Check sheet for the modelled part. Datum: model origin and axes. Units: mm. A direction names the side the tool comes from. Give positions to 0.01 mm unless a question says otherwise; leave off trailing zeros. Loops run counter-clockwise (first coordinate to the right, second up) from the corner with the lowest first, then second, coordinate; pieces in that order, holes last. Notation, with made-up numbers: M -17,81.5 L 38,81.5 A21 ccw 38,116.5 Z; hole C 71,74 d2. An arc over 180 degrees is marked long. Use one line per item in the form item = value.
from build123d import *

# Parameters (mm, degrees)
SKETCH1_W                 = 140
SKETCH1_H                 = 30
BOSS_EXTRUDE1_DEPTH       = 5
EXTRUDE_THIN1_START       = -5
EXTRUDE_THIN1_OUTLINE_W   = 20
EXTRUDE_THIN1_OUTLINE_H   = 30
EXTRUDE_THIN1_OUTLINE_W_2 = 16
EXTRUDE_THIN1_OUTLINE_H_2 = 26
EXTRUDE_THIN1_DEPTH       = 85
FILLET1_SIZE              = 15
SKETCH3_R                 = 17
SKETCH3_R_2               = 15
EXTRUDE_THIN2_DEPTH       = 40
SKETCH4_W                 = 35
SKETCH4_H                 = 24.79
BOSS_EXTRUDE2_DEPTH       = 160


with BuildPart() as part:
    # Sketch1 → Boss-Extrude1 (new body)
    with BuildSketch(Plane(origin=(0, 0, 0), x_dir=(1, 0, 0), z_dir=(0, 1, 0))):
        Rectangle(SKETCH1_W, SKETCH1_H)
    extrude(amount=-BOSS_EXTRUDE1_DEPTH)

    # Extrude-Thin1: read off the stored shape, not the designer's step
    # Extrude-Thin1 outline → Extrude-Thin1 (add)
    # profile 1 of 2: a face of its own
    with BuildSketch(Plane(origin=(0, 0, 0), x_dir=(1, 0, 0), z_dir=(0, 1, 0)).offset(EXTRUDE_THIN1_START)):
        with Locations((60, 0)):
            Rectangle(EXTRUDE_THIN1_OUTLINE_W, EXTRUDE_THIN1_OUTLINE_H)
        with Locations((60, 0)):
            Rectangle(EXTRUDE_THIN1_OUTLINE_W_2, EXTRUDE_THIN1_OUTLINE_H_2, mode=Mode.SUBTRACT)
    # profile 2 of 2: a face of its own
    with BuildSketch(Plane(origin=(0, 0, 0), x_dir=(1, 0, 0), z_dir=(0, 1, 0)).offset(EXTRUDE_THIN1_START)):
        with Locations((-60, 0)):
            Rectangle(EXTRUDE_THIN1_OUTLINE_W, EXTRUDE_THIN1_OUTLINE_H)
        with Locations((-60, 0)):
            Rectangle(EXTRUDE_THIN1_OUTLINE_W_2, EXTRUDE_THIN1_OUTLINE_H_2, mode=Mode.SUBTRACT)
    extrude(amount=EXTRUDE_THIN1_DEPTH)

    # Fillet1
    # a fillet whose section is not a circle: 15 mm, written as the material it takes off along each edge
    with BuildSketch(Plane(origin=(-107.5, 80, 15), x_dir=(0, -1, 0), z_dir=(1, 0, 0)), Plane(origin=(-12.5, 80, -15), x_dir=(0, -1, 0), z_dir=(-1, 0, 0)), Plane(origin=(107.5, 80, -15), x_dir=(0, -1, 0), z_dir=(-1, 0, 0)), Plane(origin=(12.5, 80, 15), x_dir=(0, -1, 0), z_dir=(1, 0, 0))) as fillet1_piece_1:
        with BuildLine():
            Bezier((FILLET1_SIZE, 0), (0, 0), (0, FILLET1_SIZE), weights=[1, 1.060660172, 1])
            Line((0, FILLET1_SIZE), (0, 0))
            Line((0, 0), (FILLET1_SIZE, 0))
        make_face()
    extrude(amount=95, mode=Mode.SUBTRACT)

    # Sketch3 → Extrude-Thin2 (add)
    with BuildSketch(Plane.ZY.offset(70)):
        with Locations((0, 65)):
            Circle(SKETCH3_R)
        with Locations((0, 65)):
            Circle(SKETCH3_R_2, mode=Mode.SUBTRACT)
    extrude_thin2 = extrude(amount=-EXTRUDE_THIN2_DEPTH)

    # Mirror1: Extrude-Thin2 across plane
    add(extrude_thin2.mirror(Plane(origin=(0, 0, 0), x_dir=(0, 0, 1), z_dir=(1, 0, 0))))

    # Sketch4 → Boss-Extrude2 (add)
    with BuildSketch(Plane.XZ.offset(5)):
        Rectangle(SKETCH4_W, SKETCH4_H)
    extrude(amount=BOSS_EXTRUDE2_DEPTH)


solid = part.part
1) Depth check by flat-ended pin: pin 1 Ø13 at (x, y) = (-62, 36) entering from -Z; pin 2 Ø15 at (x, z) = (-4, -3) entering from +Y; pin 3 Ø8 at (x, y) = (56, 15.5) entering from +Z. Enter the tip coordinate at first touch or a pass-through.
Evaluation:
pin_1 = -15
pin_2 = 0
pin_3 = 15
2) Release check for a two-part mould opening along X. For faces 4 (the face through (-17.5, -84, 0)), 5 (the face through (52, 27, 0)), 6 (the face through (0, -1, -15)) record: pulls with the +X half, pulls with the -X half, needs draft (parallel to the pull), parting line crosses it, or undercut.
Evaluation:
face_4 = pulls with the -X half
face_5 = undercut
face_6 = needs draft
3) Section check C-C (x = -1.5). Record the cut outline in (y, z) (3 decimals), then the cut area to 3 significant figures.
Evaluation:
outline = M -165,-12.395 L -5,-12.395 L -5,-15 L 0,-15 L 0,15 L -5,15 L -5,12.395 L -165,12.395 Z
area = 4,120 mm^2
4) Scan lines: line 1 (Y direction, x = 44.5, z = 0); line 2 (X direction, y = 51, z = -5); line 3 (Z direction, x = 42, y = 65). Record each from-to range of solid material in increasing order.
Evaluation:
line_1 = -5 to 0, 48 to 50, 80 to 82
line_2 = -70 to -68, -52 to -50, 50 to 52, 68 to 70
line_3 = -17 to -15, 15 to 17
5) Section check D-D (z = 0). State how many separate pieces and enclosed holes the cut face has, then the cut area to 3 significant figures.
Evaluation:
separate_pieces = 1
enclosed_holes = 4
area = 7,240 mm^2
6) Section check A-A (x = 58). Record the cut outline in (y, z).
Evaluation:
outline = M -5,-15 L 57,-15 A17 ccw long 57,15 L -5,15 Z; hole M 0,-13 L 54.05,-13 A17 cw 54.05,13 L 0,13 Z; hole M 57.52,-13 L 72.48,-13 A15 ccw 72.48,13 L 57.52,13 A15 ccw Z
7) Section check B-B (y = 65). Record the cut outline in (x, z), then the cut area to 3 significant figures.
Evaluation:
outline = M -70,-17 L -30,-17 L -30,-15 L -50,-15 L -50,15 L -30,15 L -30,17 L -70,17 Z; M 30,-17 L 70,-17 L 70,17 L 30,17 L 30,15 L 50,15 L 50,-15 L 30,-15 Z; hole M -68,-13 L -52,-13 L -52,13 L -68,13 Z; hole M 52,-13 L 68,-13 L 68,13 L 52,13 Z
area = 688 mm^2
8) Set-up check for faces 1 (the face through (17.5, -84, 0)), 2 (the face through (-1, 0, 0)), 3 (the face through (-60, 0, 0)): record each of +Z, -Z, +X, -X, +Y, -Y from which the full face is reachable in a straight line by a thin tool's end or side.
Evaluation:
face_1 = +Z, -Z, +X, -Y
face_2 = +Z, -Z
face_3 = none
